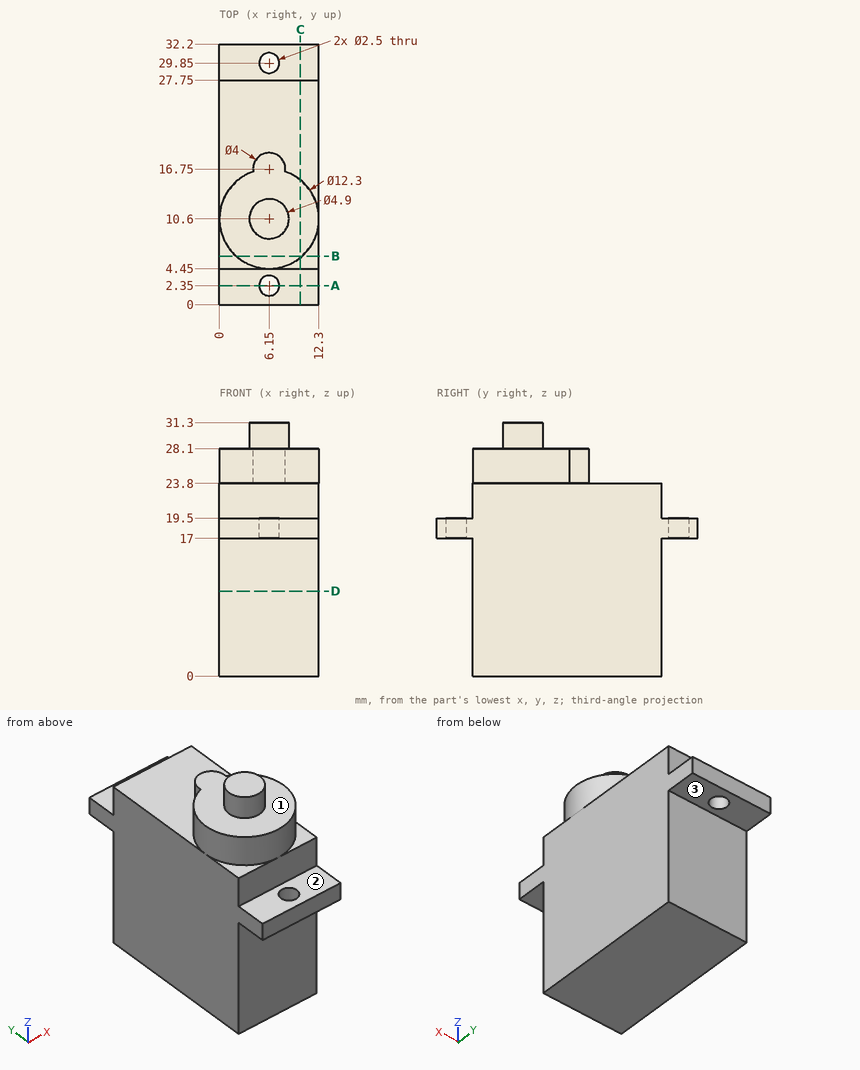
Verification items for this drawing (mm, ordinates from the low corner). A direction names the side the tool comes from. Round coordinates to 2 decimals unless told otherwise and drop trailing zeros. Order: outer loops, then holes, each group sorted by start corner. A loop starts at its lowest first (then second) coordinate and runs counter-clockwise, first axis right, second up.
1) Material ranges on line 1 (Y direction, x = 6.15, z = 18.9); line 2 (Z direction, x = 6.5, y = 5.5); line 3 (Y direction, x = 11.5, z = 11.5), recorded low to high.
Geometry says:
line 1: y = 0 to 1.1, 3.6 to 28.6, 31.1 to 32.2
line 2: z = 0 to 28.1
line 3: y = 4.45 to 27.75
2) Depth check by flat-ended pin: pin 1 (2 mm diameter, centred on x = 6.5, z = 21, fed in from -Y); pin 2 (5 mm diameter, centred on x = 5, y = 30, fed in from -Z); pin 3 (2 mm diameter, centred on x = 6.15, y = 29.85, fed in from -Z); pin 4 (3 mm diameter, centred on x = 6.15, y = 2.35, fed in from +Z). Enter the tip coordinate at first touch or a pass-through.
Geometry says:
pin 1: stops at y = 4.45
pin 2: stops at z = 0
pin 3: passes through
pin 4: stops at z = 19.5
3) Cross-section at B-B, the plane y = 6. Record the cut outline in (x, z), plus the area to 3 significant figures.
Geometry says:
outline: (0, 0) - (12.3, 0) - (12.3, 23.8) - (10.23, 23.8) - (10.23, 28.1) - (2.07, 28.1) - (2.07, 23.8) - (0, 23.8) - close
area: 328 mm2
4) Tool access check on the marked faces 1, 2 and 3. Record the directions out of +Z, -Z, +X, -X, +Y, -Y that give a thin tool (end or side, any length) a straight path to the whole face; none if there is none.
Geometry says:
face 1: +Z
face 2: +Z, +X, -X, -Y
face 3: -Z, +X, -X, +Y
5) Cross-section at A-A, the plane y = 2.35. Record the cut outline in (x, z).
Geometry says:
outline: (0, 17) - (4.9, 17) - (4.9, 19.5) - (0, 19.5) - close; (7.4, 17) - (12.3, 17) - (12.3, 19.5) - (7.4, 19.5) - close
6) Cross-section at D-D, the plane z = 10.5. Record the cut outline in (x, y).
Geometry says:
outline: (0, 4.45) - (12.3, 4.45) - (12.3, 27.75) - (0, 27.75) - close
7) Cross-section at C-C, the plane x = 10. Record the cut outline in (y, z), plus the area to 3 significant figures.
Geometry says:
outline: (0, 17) - (4.45, 17) - (4.45, 0) - (27.75, 0) - (27.75, 17) - (32.2, 17) - (32.2, 19.5) - (27.75, 19.5) - (27.75, 23.8) - (15.4, 23.8) - (15.4, 28.1) - (5.8, 28.1) - (5.8, 23.8) - (4.45, 23.8) - (4.45, 19.5) - (0, 19.5) - close
area: 618 mm2
